For this review, take the finished solid that the model builds, in its own axes (mm). A direction names the side the tool comes from. Give positions to 0.01 mm unless a question says otherwise; leave off trailing zeros. Put each result on its own line as item: value. Start each with the question number.
Autodesk Inventor part; units mm, degrees
ref_plane "Arbeitsebene2" through (-22.1367, 25.157, 0) normal (-1, 0, 0) x (0, 0, 1)
ref_plane "Arbeitsebene3" through (-21.9295, 1679.3618, 0) normal (-0.1021834, -0.9947656, 0) x (0, 0, 1)
ref_plane "Profilebene" through (14.4313, 25.2856, 0) normal (-0.0035178, 0.9999938, 0) x (0, 0, 1)
ref_plane "Arbeitsebene2" through (-22.1367, 25.157, 0) normal (-1, 0, 0) x (0, 0, 1)
ref_plane "Arbeitsebene3" through (-21.9295, 1679.3618, 0) normal (-0.1021834, -0.9947656, 0) x (0, 0, 1)
sketch "Pfad" plane through (0, 0, 0) normal (0, 0, 1) x (1, 0, 0)
  arc A0 (-58.7046, 25.2948) -> (14.4313, 25.2856) centre (-22.1367, 25.157) ccw
  arc A1 (8.6121, 1679.4693) -> (-52.4711, 1679.4769) centre (-21.9295, 1679.3618) ccw
  line L0 (8.6121, 1679.4693) -> (14.4313, 25.2856)
  line L1 (-58.7046, 25.2948) -> (-52.4711, 1679.4769)
  dimension "d31" = 11.9888
ref_plane "Profilebene" through (14.4313, 25.2856, 0) normal (-0.0035178, 0.9999938, 0) x (0, 0, 1)
sketch "Profilskizze" plane through (14.4313, 25.2856, 0) normal (-0.0035178, 0.9999938, 0) x (0, 0, 1)
  line L0 (-8.509, -1.9812) -> (8.509, -1.9812)
  line L1 (8.509, -1.9812) -> (8.509, 1.9812)
  line L2 (8.509, 1.9812) -> (-8.509, 1.9812)
  line L3 (-8.509, 1.9812) -> (-8.509, -1.9812)
  line L4 (-3.9624, -3.9624) -> (3.9624, -3.9624)
  line L5 (3.9624, -3.9624) -> (3.9624, 3.9624)
  line L6 (3.9624, 3.9624) -> (-3.9624, 3.9624)
  line L7 (-3.9624, 3.9624) -> (-3.9624, -3.9624)
  line L8 (-3.9624, 0) -> (3.9624, 0) construction
  line L9 (-7.0104, -5.9944) -> (-3.9624, -5.9944)
  line L10 (-3.9624, -5.9944) -> (-3.9624, 5.9944)
  line L11 (-3.9624, 5.9944) -> (-7.0104, 5.9944)
  line L12 (-7.0104, 5.9944) -> (-7.0104, -5.9944)
  line L13 (3.9624, -5.9944) -> (7.0104, -5.9944)
  line L14 (7.0104, -5.9944) -> (7.0104, 5.9944)
  line L15 (7.0104, 5.9944) -> (3.9624, 5.9944)
  line L16 (3.9624, 5.9944) -> (3.9624, -5.9944)
  line L17 (-8.509, 0) -> (8.509, 0) construction
  point P0 (0, 0)
  point P1 (0, 0)
  dimension "d21" = 3.9624
  dimension "d22" = 7.9248
  dimension "d23" = 7.9248
  dimension "d24" = 3.048
  dimension "d31" = 11.9888
  dimension "d32" = 17.018
sweep "Volumenkörper" add profiles "Profilskizze" path "Pfad"
pattern_of_one "Strand Pattern"
equation "\"d21\" = da_d2"
equation "\"d22\" = da_d1"
equation "\"d23\" = da_b1"
equation "\"d24\" = da_t1 + da_t2"
equation "\"d30\" = da_pt"
equation "\"da_p\" = 12.7"
equation "\"da_b1\" = 7.9248"
equation "\"da_h2\" = 11.9888"
equation "\"da_h3\" = 10.3886"
equation "\"da_d1\" = 7.9248"
equation "\"da_d2\" = 3.9624"
equation "\"da_pt\" = 14.3764"
equation "\"da_b\" = 17.018"
equation "\"da_t1\" = 1.524"
equation "\"da_t2\" = 1.524"
properties part number "HTW-000643" material "Edelstahl"
1. Wall thickness on line 1 (Z direction, x = 6.5, y = 703); line 2 (X direction, y = 630, z = -7.5); line 3 (X direction, y = 1172.5, z = 1.75): over which ranges is each line inside the solid? List them lowest first. Write a range as from..to.
2. The part is to be moulded in two halves that separate along Y. For faces 5 (the face through (-22.639, 1711.877, 7.749)), 6 (the face through (-21.299, 1707.915, 7.77)), 7 (the face through (-22.86, -7.44, 0.06)), 8 (the face through (16, 845, -7.01)), say which applies: released by +Y, released by -Y, zero draft, split by the parting line, or undercut.
3. Tool access review of faces 1 (the face through (-22.682, 1713.858, -0.055)), 2 (the face through (-21.299, 1707.915, -7.749)), 3 (the face through (-22.81, -5.41, -5.47)), 4 (the face through (-51, 845, 3.962)): name each direction out of +Z, -Z, +X, -X, +Y, -Y from which nothing blocks a thin tool from reaching the whole face with its end or side.
4. Clearance check with flat-ended pins moving along their axes: pin 1 (1 mm diameter, centred on x = -53.5, y = 344.5, fed in from +Z); pin 2 (6 mm diameter, centred on x = -5, z = 3, fed in from -Y); pin 3 (5 mm diameter, centred on x = -53.5, z = 2.5, fed in from -Y). State where each tip first meets the part, or that it passes through.
Found:
1. line 1: z = -7.01..-3.96, 3.96..7.01
1. line 2: x = -58.41..-54.44, 10.32..14.29
1. line 3: x = -58.34..-50.42, 6.43..14.36
2. face 5: released by +Y
2. face 6: undercut
2. face 7: undercut
2. face 8: zero draft
3. face 1: +Y
3. face 2: -Z
3. face 3: +Z, -Z
3. face 4: none
4. pin 1: stops at z = 7.01
4. pin 2: stops at y = -14.93
4. pin 3: stops at y = -5.68
